CAD build for the part. Positions are in the model's coordinates, mm. A direction names the side the tool comes from. Give positions to 0.01 mm unless a question says otherwise; leave off trailing zeros. Loops run counter-clockwise (first coordinate to the right, second up) from the corner with the lowest first, then second, coordinate; pieces in that order, holes last.
```python
from build123d import *

# Parameters (mm, degrees)
BOSS_EXTRUDE1_DEPTH = 4.5
SKETCH2_R           = 4
SKETCH2_R_2         = 2.5
CUT_EXTRUDE1_DEPTH  = 9
SKETCH3_R           = 2
CUT_EXTRUDE2_DEPTH  = 26.154522456
CHAMFER1_SIZE       = 1


with BuildPart() as part:
    # Sketch1 → Boss-Extrude1 (new, symmetric)
    with BuildSketch(Plane.XY):
        with BuildLine():
            Line((6, 16.439282223), (6, 5))
            ThreePointArc((6, 5), (7.464466094, 1.464466094), (11, 0))
            Line((11, 0), (17.5, 0))
            ThreePointArc((17.5, 0), (0, -17.5), (-17.5, 0))
            Line((-17.5, 0), (-11, 0))
            ThreePointArc((-11, 0), (-7.464466094, 1.464466094), (-6, 5))
            Line((-6, 5), (-6, 16.439282223))
            ThreePointArc((-6, 16.439282223), (0, 17.5), (6, 16.439282223))
        make_face()
    extrude(amount=BOSS_EXTRUDE1_DEPTH, both=True)

    # Sketch2 → Cut-Extrude1 (cut)
    with BuildSketch(Plane.XY.offset(4.5)):
        Circle(SKETCH2_R)
        with Locations((0, 12.7)):
            Circle(SKETCH2_R_2)
    extrude(amount=-CUT_EXTRUDE1_DEPTH, mode=Mode.SUBTRACT)

    # Sketch3 → Cut-Extrude2 (cut, through all)
    with BuildSketch(Plane(origin=(0, 0, 0), x_dir=(1, 0, 0), z_dir=(0, 1, 0))):
        with Locations(Location((0, 0, 0), (0, 0, 270))):
            Circle(SKETCH3_R)
    extrude(amount=-CUT_EXTRUDE2_DEPTH, mode=Mode.SUBTRACT)

    # Chamfer1
    chamfer1_edges = [part.edges().sort_by_distance(p)[0] for p in [
        (0, 17.5, -4.5),
        (0, -17.5, 4.5),
        (0, 17.5, 4.5),
        (0, -17.5, -4.5),
    ]]
    chamfer(chamfer1_edges, length=CHAMFER1_SIZE)


solid = part.part
```
1. Saw through at C-C, the plane z = -0.25. List the corners of the cut face in (x, y), and give its area (3 significant figures).
Responses:
outline: (-17.5, 0) arc R17.5 ccw to (-1.98, -17.39) - (-1.98, -3.47) arc R4 cw (long way) to (1.98, -3.47) - (1.98, -17.39) arc R17.5 ccw to (17.5, 0) - (11, 0) arc R5 cw to (6, 5) - (6, 16.44) arc R17.5 ccw to (-6, 16.44) - (-6, 5) arc R5 cw to (-11, 0) - close; hole circle Ø5 at (0, 12.7)
area: 574 mm2
2. Saw through at A-A, the plane y = 12.7. List the corners of the cut face in (x, z).
Responses:
outline: (-6, -4.5) - (-2.5, -4.5) - (-2.5, 4.5) - (-6, 4.5) - close; (2.5, -4.5) - (6, -4.5) - (6, 4.5) - (2.5, 4.5) - close
3. Tool access for faces 1 (the face through (14, 0, 0)), 2 (the face through (-6, 11, 0)), 3 (the face through (-2, -10, 0)): list every direction of +Z, -Z, +X, -X, +Y, -Y with a clear straight run to the whole face (end or side of a thin tool).
Responses:
face 1: +Z, -Z, +X, +Y
face 2: +Z, -Z, -X, +Y
face 3: -Y
4. Drop flat-ended pins along their axis: pin 1 (4 mm diameter, centred on y = -4, z = 1.5, fed in from +X); pin 2 (5 mm diameter, centred on x = 14.5, z = 0, fed in from +Y); pin 3 (1.5 mm diameter, centred on y = -4, z = 3, fed in from +X). Give the stop position or say it passes through.
Responses:
pin 1: stops at x = 17.39
pin 2: stops at y = 0
pin 3: stops at x = 17.2
5. Saw through at D-D, the plane y = 9. List the corners of the cut face in (x, z).
Responses:
outline: (-6, -4.5) - (6, -4.5) - (6, 4.5) - (-6, 4.5) - close
6. Probe line 1 along Z through (x, y) = (0, -13); line 2 along Y through (x, z) = (0, -0.25); line 3 along X through (y, z) = (-4.5, -1.5). List the from-to ranges inside material, lowest first.
Responses:
line 1: z = -4.5 to -2, 2 to 4.5
line 2: y = 4 to 10.2, 15.2 to 17.5
line 3: x = -16.91 to -1.32, 1.32 to 16.91
7. Saw through at B-B, the plane z = 2.75. List the corners of the cut face in (x, y), and give its area (3 significant figures).
Responses:
outline: (-17.5, 0) arc R17.5 ccw to (17.5, 0) - (11, 0) arc R5 cw to (6, 5) - (6, 16.44) arc R17.5 ccw to (-6, 16.44) - (-6, 5) arc R5 cw to (-11, 0) - close; hole circle Ø8 at (0, 0); hole circle Ø5 at (0, 12.7)
area: 628 mm2
8. Pull direction X, two halves, no side cores. Call faces 4 (the face through (0, -7, 4.5)), 5 (the face through (-0.521, 3.966, 0.063)), 6 (the face through (0, 17, 4)), 7 (the face through (-0.33, 15.18, 0.06)): released by +X, released by -X, zero draft, split by the parting line, or undercut.
Responses:
face 4: zero draft
face 5: undercut
face 6: split by the parting line
face 7: undercut
